```python
from build123d import *

# Parameters (mm, degrees)
SKETCH1_W           = 75
SKETCH1_H           = 100
SKETCH1_R           = 2
SKETCH1_R_2         = 2.75
BOSS_EXTRUDE1_DEPTH = 10


with BuildPart() as part:
    # Sketch1 → Boss-Extrude1 (new body)
    with BuildSketch(Plane.XY):
        with Locations((-37.5, 0)):
            Rectangle(SKETCH1_W, SKETCH1_H)
        with Locations((-40.75, 37.5)):
            Circle(SKETCH1_R, mode=Mode.SUBTRACT)
        with Locations((-9.25, 37.5)):
            Circle(SKETCH1_R, mode=Mode.SUBTRACT)
        with Locations((-40.75, 11.5)):
            Circle(SKETCH1_R, mode=Mode.SUBTRACT)
        with Locations((-9.25, 11.5)):
            Circle(SKETCH1_R, mode=Mode.SUBTRACT)
        with Locations((-40.75, -11.5)):
            Circle(SKETCH1_R, mode=Mode.SUBTRACT)
        with Locations((-9.25, -11.5)):
            Circle(SKETCH1_R, mode=Mode.SUBTRACT)
        with Locations((-9.25, -37.5)):
            Circle(SKETCH1_R, mode=Mode.SUBTRACT)
        with Locations((-40.75, -37.5)):
            Circle(SKETCH1_R, mode=Mode.SUBTRACT)
        with Locations((-60.75, 41.904631992)):
            Circle(SKETCH1_R_2, mode=Mode.SUBTRACT)
        with Locations((-60.75, 9.904631992)):
            Circle(SKETCH1_R_2, mode=Mode.SUBTRACT)
        with Locations((-60.75, -9.904631992)):
            Circle(SKETCH1_R_2, mode=Mode.SUBTRACT)
        with Locations((-60.75, -41.904631992)):
            Circle(SKETCH1_R_2, mode=Mode.SUBTRACT)
    extrude(amount=BOSS_EXTRUDE1_DEPTH)


solid = part.part
```
Design review of the part built by this model. Coordinates are the model's own, in mm. Give positions to 0.01 mm unless a question says otherwise; leave off trailing zeros. Order: outer loops, then holes, each group sorted by start corner. A loop starts at its lowest first (then second) coordinate and runs counter-clockwise, first axis right, second up. Notation, with made-up numbers: M 22,-26.75 L 59,-26.75 A26 ccw 59,-7.75 Z; hole C -3,50.5 d6. An arc over 180 degrees is marked long. One line per question, with ' | ' between items. Start each with the question number.
Q1. The part is to be moulded in two halves that separate along Y. For faces 1 (the face through (-38, 50, 5)), 2 (the face through (-41.184, 35.548, 4.93)), 3 (the face through (-75, -1, 5)), 4 (the face through (-41.01, 13.483, 4.93)), say which applies: +Y half, -Y half, draft (parallel to the pull), parting line (faces both ways), or undercut.
Q2. We need section D-D (y = 11.5). Write out the cut boundary in (x, z), plus the area to 3 significant figures.
Q3. For pin 1 Ø3.5 at (x, y) = (-60.75, -9.9) entering from -Z, flat-tipped, find the tip position at first contact; note if it passes through.
Q4. We need section C-C (z = 7.75). State how many separate pieces and enclosed holes the cut face has, plus the area to 3 significant figures.
Q5. For L1, parallel to Y at x = -40.75, z = 3.5; L2, parallel to Y at x = -60.75, z = 4.5; L3, parallel to X at y = 42.5, z = 0.5, list the stretches that pass through material, from the lowest coordinate up. Write a range as [from, to].
Q6. We need section A-A (x = -60.75). Write out the cut boundary in (y, z), plus the area to 3 significant figures.
Q7. We need section B-B (y = -37.5). Write out the cut boundary in (x, z).
Returned:
1) face 1: +Y half | face 2: undercut | face 3: draft | face 4: undercut
2) outline: M -75,0 L -62.99,0 L -62.99,10 L -75,10 Z; M -58.51,0 L -42.75,0 L -42.75,10 L -58.51,10 Z; M -38.75,0 L -11.25,0 L -11.25,10 L -38.75,10 Z; M -7.25,0 L 0,0 L 0,10 L -7.25,10 Z | area: 625 mm2
3) pin 1: through
4) separate pieces: 1 | enclosed holes: 12 | area: 7,300 mm2
5) L1: [-50, -39.5], [-35.5, -13.5], [-9.5, 9.5], [13.5, 35.5], [39.5, 50] | L2: [-50, -44.65], [-39.15, -12.65], [-7.15, 7.15], [12.65, 39.15], [44.65, 50] | L3: [-75, -63.43], [-58.07, 0]
6) outline: M -50,0 L -44.65,0 L -44.65,10 L -50,10 Z; M -39.15,0 L -12.65,0 L -12.65,10 L -39.15,10 Z; M -7.15,0 L 7.15,0 L 7.15,10 L -7.15,10 Z; M 12.65,0 L 39.15,0 L 39.15,10 L 12.65,10 Z; M 44.65,0 L 50,0 L 50,10 L 44.65,10 Z | area: 780 mm2
7) outline: M -75,0 L -42.75,0 L -42.75,10 L -75,10 Z; M -38.75,0 L -11.25,0 L -11.25,10 L -38.75,10 Z; M -7.25,0 L 0,0 L 0,10 L -7.25,10 Z
